```python
from build123d import *

# Parameters (mm, degrees)
SKETCH1_R           = 13
BOSS_EXTRUDE1_DEPTH = 20
CHAMFER1_SIZE       = 3
CHAMFER2_SIZE       = 1
SKETCH2_R           = 2.75
CUT_EXTRUDE1_DEPTH  = 21
CUT_EXTRUDE2_REACH  = 45
SKETCH3_R           = 3.3
SKETCH4_R           = 5.4
CUT_EXTRUDE3_DEPTH  = 1.5
CHAMFER3_SIZE       = 0.5
FILLET1_R           = 0.3


with BuildPart() as part:
    # Sketch1 → Boss-Extrude1 (new body)
    with BuildSketch(Plane.XY):
        Polygon((17, 0), (-17, 0), (-17, -10.5), (-30, -10.5), (-30, -43), (30, -43), (30, -10.5), (17, -10.5), align=None)
        with Locations((0, -18)):
            Circle(SKETCH1_R, mode=Mode.SUBTRACT)
    extrude(amount=BOSS_EXTRUDE1_DEPTH)

    # Chamfer1
    chamfer1_edges = [part.edges().sort_by_distance(p)[0] for p in [
        (-17, 0, 10),
        (17, 0, 10),
    ]]
    chamfer(chamfer1_edges, length=CHAMFER1_SIZE)

    # Chamfer2
    chamfer2_edges = [part.edges().sort_by_distance(p)[0] for p in [
        (23.5, -10.5, 20),
        (30, -26.75, 0),
        (0, -43, 0),
        (17, -6.75, 20),
        (-30, -43, 10),
        (-30, -10.5, 10),
        (30, -10.5, 10),
        (30, -43, 10),
        (-13, -18, 0),
        (-13, -18, 20),
        (-23.5, -10.5, 20),
        (-30, -26.75, 20),
        (0, 0, 0),
        (0, 0, 20),
        (-17, -6.75, 0),
        (-15.5, -1.5, 0),
        (15.5, -1.5, 0),
        (-17, -6.75, 20),
        (-15.5, -1.5, 20),
        (15.5, -1.5, 20),
        (0, -43, 20),
        (30, -26.75, 20),
        (-30, -26.75, 0),
        (-23.5, -10.5, 0),
        (17, -6.75, 0),
        (23.5, -10.5, 0),
    ]]
    chamfer(chamfer2_edges, length=CHAMFER2_SIZE)

    # Sketch2 → Cut-Extrude1 (cut, through all)
    with BuildSketch(Plane(origin=(0, 0, 0), x_dir=(-1, 0, 0), z_dir=(0, 0, -1))):
        with Locations((-23, -18)):
            Circle(SKETCH2_R)
        with Locations((23, -18)):
            Circle(SKETCH2_R)
        with Locations((23, -36)):
            Circle(SKETCH2_R)
        with Locations((-23, -36)):
            Circle(SKETCH2_R)
    extrude(amount=-CUT_EXTRUDE1_DEPTH, mode=Mode.SUBTRACT)

    # Sketch3 → Cut-Extrude2 (cut, up to next)
    with BuildSketch(Plane.XZ.offset(43), mode=Mode.PRIVATE) as cut_extrude2_sk1:
        with Locations((23, 10)):
            Circle(SKETCH3_R)
    cut_extrude2_tool1 = extrude(cut_extrude2_sk1.sketch, amount=-CUT_EXTRUDE2_REACH, mode=Mode.PRIVATE) & part.part
    add(cut_extrude2_tool1.solids().sort_by_distance((23, -43, 10))[0], mode=Mode.SUBTRACT)
    # Sketch3 → Cut-Extrude2 (cut, up to next)
    with BuildSketch(Plane.XZ.offset(43), mode=Mode.PRIVATE) as cut_extrude2_sk2:
        with Locations((-23, 10)):
            Circle(SKETCH3_R)
    cut_extrude2_tool2 = extrude(cut_extrude2_sk2.sketch, amount=-CUT_EXTRUDE2_REACH, mode=Mode.PRIVATE) & part.part
    add(cut_extrude2_tool2.solids().sort_by_distance((-23, -43, 10))[0], mode=Mode.SUBTRACT)

    # Sketch4 → Cut-Extrude3 (cut)
    with BuildSketch(Plane(origin=(0, -10.5, 0), x_dir=(1, 0, 0), z_dir=(0, 1, 0))):
        with Locations((23, -10)):
            Circle(SKETCH4_R)
        with Locations((-23, -10)):
            Circle(SKETCH4_R)
    extrude(amount=-CUT_EXTRUDE3_DEPTH, mode=Mode.SUBTRACT)

    # Chamfer3
    chamfer3_edges = [part.edges().sort_by_distance(p)[0] for p in [
        (25.75, -18, 20),
        (25.75, -18, 0),
        (-20.25, -18, 20),
        (-20.25, -18, 0),
        (-20.25, -36, 20),
        (-20.25, -36, 0),
        (25.75, -36, 20),
        (25.75, -36, 0),
        (19.7, -43, 10),
        (-26.3, -43, 10),
    ]]
    chamfer(chamfer3_edges, length=CHAMFER3_SIZE)

    # Fillet1
    fillet1_edges = [part.edges().sort_by_distance(p)[0] for p in [
        (17.6, -10.5, 10),
        (-28.4, -10.5, 10),
    ]]
    fillet(fillet1_edges, radius=FILLET1_R)


solid = part.part
```
Input: part model. Units: mm. Frame: model coordinates. A direction names the side the tool comes from. Give positions to 0.01 mm unless a question says otherwise; leave off trailing zeros. Order: outer loops, then holes, each group sorted by start corner. A loop starts at its lowest first (then second) coordinate and runs counter-clockwise, first axis right, second up. Notation, with made-up numbers: (68, 15) -> (83, 15) arc R27 cw to (83, 41) -> close; hole circle Ø5 at (-1.75, -8). An arc over 180 degrees is marked (long way). Write each question's results on one line, items separated by ' | '. Start each with the question number.
Item 1: Cut plane A-A on x = 0. Return the cut outline in (y, z), then the cut area to 3 significant figures.
Item 2: Mould query, pull axis Y, two halves, no side actions, for faces 1 (the flat face through (-30, -27, 10)), 2 (the cylindrical face through (-25.62, -35.17, 15.61)), 3 (the flat face through (16, -2, 10)). Classes: pulls with the +Y half, pulls with the -Y half, needs draft (parallel to the pull), parting line crosses it, or undercut.
Item 3: Cut plane B-B on y = -36. Give the number of separate pieces and of enclosed holes in the cut face, then the cut area to 3 significant figures.
Item 4: Cut plane C-C on z = 17. Return the cut outline in (x, y).
Item 5: Contact query for flat-ended pins moving along their axis: P1, Ø6, axis at y = -5.5, z = 12, coming from the +X side; P2, Ø5.5, axis at x = -21.5, z = 8, coming from the +Y side; P3, Ø7.5, axis at x = -23, z = 10, coming from the -Y side. Output: stop coordinate, or through.
Item 6: Set-up query: faces 4 (the flat face through (23, -12, 14)), 5 (the flat face through (-23, -10.5, 4)), 6 (the flat face through (23, -10.5, 4)), 7 (the flat face through (15.12, -1.84, 19.51)), 8 (the flat face through (0, -35, 0)). Return all of +Z, -Z, +X, -X, +Y, -Y with unobstructed straight access to the full face (end or side cutting, diameter ignored); none if empty.
Item 7: Line query: line 1 (Y direction, x = 23, z = 5); line 2 (Y direction, x = 23, z = 16.75); line 3 (X direction, y = -36, z = 18). Output: solid intervals per line, ascending.
Established:
1) outline: (-43, 1) -> (-42, 0) -> (-32, 0) -> (-31, 1) -> (-31, 19) -> (-32, 20) -> (-42, 20) -> (-43, 19) -> close; (-5, 1) -> (-4, 0) -> (-1, 0) -> (0, 1) -> (0, 19) -> (-1, 20) -> (-4, 20) -> (-5, 19) -> close | area: 336 mm^2
2) face 1: needs draft | face 2: undercut | face 3: pulls with the +Y half
3) separate pieces: 3 | enclosed holes: 0 | area: 972 mm^2
4) outline: (-30, -42) -> (-29, -43) -> (29, -43) -> (30, -42) -> (30, -11.5) -> (29, -10.5) -> (17, -10.5) -> (17, -3) -> (14, 0) -> (-14, 0) -> (-17, -3) -> (-17, -10.5) -> (-29, -10.5) -> (-30, -11.5) -> close; hole circle Ø5.5 at (-23, -36); hole circle Ø5.5 at (-23, -18); hole circle Ø26 at (0, -18); hole circle Ø5.5 at (23, -36); hole circle Ø5.5 at (23, -18)
5) P1: x = 17 | P2: y = -12 | P3: y = -42.95
6) face 4: +Y | face 5: +Z, -Z, -X, +Y | face 6: +Z, -Z, +X, +Y | face 7: +Z, +X, +Y | face 8: -Z, +X, -X, +Y, -Y
7) line 1: -43 to -38.75, -33.25 to -20.75, -15.25 to -12 | line 2: -43 to -38.75, -33.25 to -20.75, -15.25 to -10.5 | line 3: -30 to -25.75, -20.25 to 20.25, 25.75 to 30
